The figure shows three views and two pictorial views of one solid part (mm, origin at its lowest corner). Answer the questions. A direction names the side the tool comes from. Round coordinates to 2 decimals unless told otherwise and drop trailing zeros. Loops run counter-clockwise (first coordinate to the right, second up) from the corner with the lowest first, then second, coordinate; pieces in that order, holes last. Notation, with made-up numbers: (4.5, -7) -> (51.5, -7) arc R17 ccw to (51.5, -2) -> close; hole circle Ø3 at (-38.75, 73.5). An arc over 180 degrees is marked (long way). Write item = value, one per line. Start each with the question number.
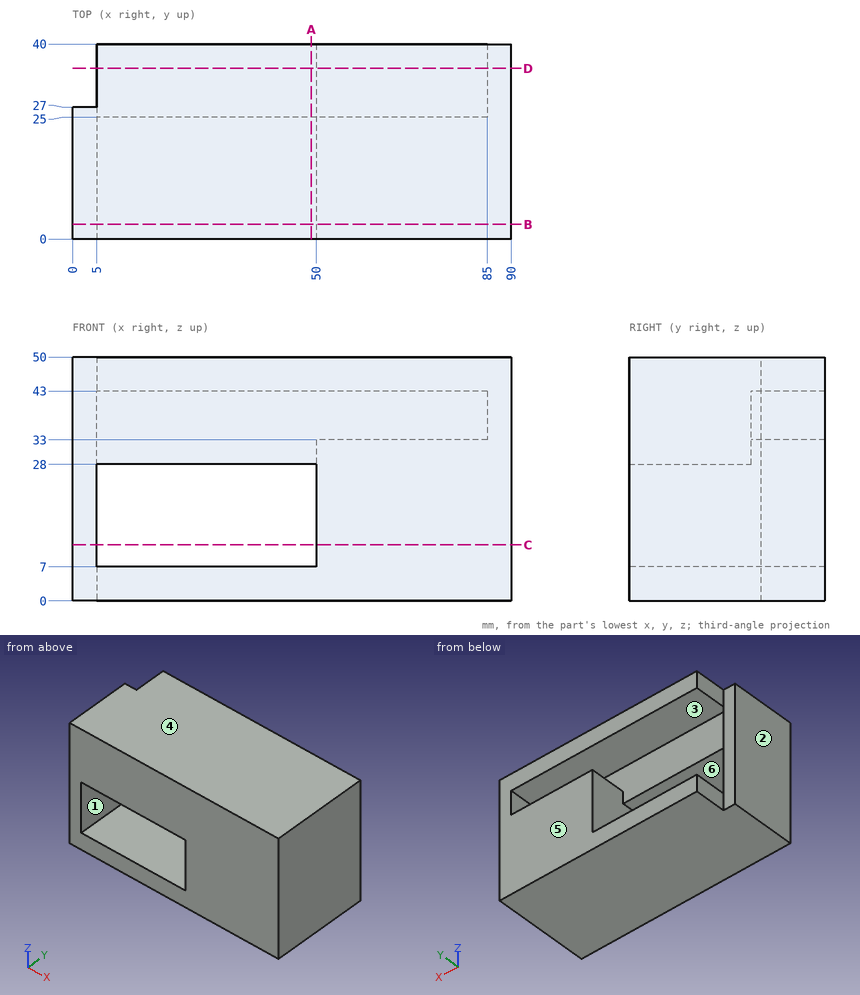
Item 1: A tool of negligible diameter and unlimited length cuts with its end or side. For the marked faces 5 and 6, from which of +Z, -Z, +X, -X, +Y, -Y can it reach the whole face along a straight path? Write none if from no direction.
Item 2: Flat-ended cylindrical pins translate along their axes: pin 1 (2 mm diameter, centred on y = 32.5, z = 48, fed in from -X); pin 2 (4.5 mm diameter, centred on x = 50.5, y = 29, fed in from -Z); pin 3 (7.5 mm diameter, centred on x = 49, z = 37.5, fed in from +Y); pin 4 (3 mm diameter, centred on y = 36, z = 36.5, fed in from -X). Find the tip coordinate at first contact, or state that the pin passes through.
Item 3: Section A-A (x = 49) is taken. Determine the outline of the cut face in (y, z).
Item 4: Section D-D (y = 35) is taken. Determine the outline of the cut face in (x, z).
Item 5: The mould has two halves that part along Z. Classify the marked faces 1, 2, 3 and 4: pulls with the +Z half, pulls with the -Z half, needs draft (parallel to the pull), parting line crosses it, or undercut.
Item 6: Section B-B (y = 3) is taken. Determine the outline of the cut face in (x, z), then the cut area to 4 significant figures.
Item 7: Find the intervals of material crossed by line 1 along Z through (x, y) = (38.5, 33.5); line 2 along Z through (x, y) = (9.5, 11); line 3 along X through (y, z) = (7, 26), in increasing order. Write a range as [from, to].
Item 8: Section C-C (z = 11.5) is taken. Determine the outline of the cut face in (x, y).
Worked answers:
q1.face_5 = +Z, -Z, +X, -X, +Y
q1.face_6 = +Y, -Y
q2.pin_1 = 5
q2.pin_2 = 0
q2.pin_3 = 25
q2.pin_4 = 85
q3.outline = (0, 0) -> (40, 0) -> (40, 7) -> (0, 7) -> close; (0, 28) -> (25, 28) -> (25, 43) -> (40, 43) -> (40, 50) -> (0, 50) -> close
q4.outline = (5, 0) -> (90, 0) -> (90, 50) -> (5, 50) -> (5, 43) -> (85, 43) -> (85, 33) -> (50, 33) -> (50, 7) -> (5, 7) -> close
q5.face_1 = undercut
q5.face_2 = needs draft
q5.face_3 = undercut
q5.face_4 = pulls with the +Z half
q6.outline = (0, 0) -> (90, 0) -> (90, 50) -> (0, 50) -> close; hole (5, 7) -> (50, 7) -> (50, 28) -> (5, 28) -> close
q6.area = 3,555 mm2
q7.line_1 = [0, 7], [43, 50]
q7.line_2 = [0, 7], [28, 50]
q7.line_3 = [0, 5], [50, 90]
q8.outline = (0, 0) -> (5, 0) -> (5, 27) -> (0, 27) -> close; (50, 0) -> (90, 0) -> (90, 40) -> (50, 40) -> close
